```python
from build123d import *

# Parameters (mm, degrees)
ESQUISSE2_W                   = 150
ESQUISSE2_H                   = 150
BOSS_EXTRU_1_DEPTH            = 35
ESQUISSE3_R                   = 42.75
ENL_V_MAT_EXTRU_2_DEPTH       = 40
ESQUISSE5_R                   = 6
ENL_V_MAT_EXTRU_3_DEPTH       = 40
ESQUISSE6_R                   = 9.5
ENL_V_MAT_EXTRU_4_DEPTH       = 13
ESQUISSE7_R                   = 5.25
ENL_V_MAT_EXTRU_5_DEPTH       = 40
ESQUISSE8_R                   = 8.5
ENL_V_MAT_EXTRU_6_DEPTH       = 11
ESQUISSE9_R                   = 4.25
ENL_V_MAT_EXTRU_7_DEPTH       = 25
ENL_V_MAT_EXTRU_8_DEPTH       = 1
ENL_V_MAT_EXTRU_8_DEPTH_BACK  = 36
ENL_V_MAT_EXTRU_12_DEPTH      = 1
ENL_V_MAT_EXTRU_12_DEPTH_BACK = 36
ENL_V_MAT_EXTRU_13_DEPTH      = 1
ENL_V_MAT_EXTRU_13_DEPTH_BACK = 36
ENL_V_MAT_EXTRU_14_DEPTH      = 1
ENL_V_MAT_EXTRU_14_DEPTH_BACK = 36
CONG_1_R                      = 10
CONG_2_R                      = 10
CONG_3_R                      = 10
CONG_4_R                      = 10
CONG_5_R                      = 2


with BuildPart() as part:
    # Esquisse2 → Boss.-Extru.1 (new body)
    with BuildSketch(Plane.XY):
        with Locations((-75, 75)):
            Rectangle(ESQUISSE2_W, ESQUISSE2_H)
    extrude(amount=BOSS_EXTRU_1_DEPTH)

    # Esquisse3 → Enlèv. mat.-Extru.2 (cut)
    with BuildSketch(Plane.XY.offset(35)):
        with Locations((-75, 75)):
            Circle(ESQUISSE3_R)
    extrude(amount=-ENL_V_MAT_EXTRU_2_DEPTH, mode=Mode.SUBTRACT)

    # Esquisse5 → Enlèv. mat.-Extru.3 (cut)
    with BuildSketch(Plane.XY.offset(35)):
        with Locations((-28.5, 101.5)):
            Circle(ESQUISSE5_R)
        with Locations((-28.5, 48.5)):
            Circle(ESQUISSE5_R)
        with Locations((-121.5, 48.5)):
            Circle(ESQUISSE5_R)
        with Locations((-121.5, 101.5)):
            Circle(ESQUISSE5_R)
    extrude(amount=-ENL_V_MAT_EXTRU_3_DEPTH, mode=Mode.SUBTRACT)

    # Esquisse6 → Enlèv. mat.-Extru.4 (cut)
    with BuildSketch(Plane.XY.offset(35)):
        with Locations((-28.5, 101.5)):
            Circle(ESQUISSE6_R)
        with Locations((-28.5, 48.5)):
            Circle(ESQUISSE6_R)
        with Locations((-121.5, 48.5)):
            Circle(ESQUISSE6_R)
        with Locations((-121.5, 101.5)):
            Circle(ESQUISSE6_R)
    extrude(amount=-ENL_V_MAT_EXTRU_4_DEPTH, mode=Mode.SUBTRACT)

    # Esquisse7 → Enlèv. mat.-Extru.5 (cut)
    with BuildSketch(Plane.XY.offset(35)):
        with Locations((-11, 139)):
            Circle(ESQUISSE7_R)
        with Locations((-11, 11)):
            Circle(ESQUISSE7_R)
        with Locations((-139, 11)):
            Circle(ESQUISSE7_R)
        with Locations((-139, 139)):
            Circle(ESQUISSE7_R)
    extrude(amount=-ENL_V_MAT_EXTRU_5_DEPTH, mode=Mode.SUBTRACT)

    # Esquisse8 → Enlèv. mat.-Extru.6 (cut)
    with BuildSketch(Plane.XY.offset(35)):
        with Locations((-11, 139)):
            Circle(ESQUISSE8_R)
        with Locations((-11, 11)):
            Circle(ESQUISSE8_R)
        with Locations((-139, 11)):
            Circle(ESQUISSE8_R)
        with Locations((-139, 139)):
            Circle(ESQUISSE8_R)
    extrude(amount=-ENL_V_MAT_EXTRU_6_DEPTH, mode=Mode.SUBTRACT)

    # Esquisse9 → Enlèv. mat.-Extru.7 (cut)
    with BuildSketch(Plane(origin=(0, 150, 0), x_dir=(1, 0, 0), z_dir=(0, 1, 0))):
        with Locations(Location((-25, -25, 0), (0, 0, 270))):  # turned: the seam where the file's is
            Circle(ESQUISSE9_R)
        with Locations(Location((-125, -25, 0), (0, 0, 270))):  # turned: the seam where the file's is
            Circle(ESQUISSE9_R)
    extrude(amount=-ENL_V_MAT_EXTRU_7_DEPTH, mode=Mode.SUBTRACT)

    # Esquisse19 → Enlèv. mat.-Extru.8 (cut, two sides)
    with BuildSketch(Plane.XY.offset(35)) as enl_v_mat_extru_8_sk:
        with BuildLine():
            Line((206.944620495, 443.229107967), (0, 115))
            ThreePointArc((0, 115), (-11.557112298, 75), (0, 35))
            Line((0, 35), (206.944620495, -293.229107967))
            Line((206.944620495, -293.229107967), (982.986947353, -293.229107967))
            Line((982.986947353, -293.229107967), (982.986947353, 443.229107967))
            Line((982.986947353, 443.229107967), (206.944620495, 443.229107967))
        make_face()
    extrude(amount=ENL_V_MAT_EXTRU_8_DEPTH, mode=Mode.SUBTRACT)
    extrude(enl_v_mat_extru_8_sk.sketch, amount=-ENL_V_MAT_EXTRU_8_DEPTH_BACK, mode=Mode.SUBTRACT)

    # Esquisse22 → Enlèv. mat.-Extru.12 (cut, two sides)
    with BuildSketch(Plane.XY.offset(35)) as enl_v_mat_extru_12_sk:
        with BuildLine():
            Line((-443.229107967, -206.944620495), (-115, 0))
            ThreePointArc((-115, 0), (-75, 11.557112298), (-35, 0))
            Line((-35, 0), (293.229107967, -206.944620495))
            Line((293.229107967, -206.944620495), (293.229107967, -982.986947353))
            Line((293.229107967, -982.986947353), (-443.229107967, -982.986947353))
            Line((-443.229107967, -982.986947353), (-443.229107967, -206.944620495))
        make_face()
    extrude(amount=ENL_V_MAT_EXTRU_12_DEPTH, mode=Mode.SUBTRACT)
    extrude(enl_v_mat_extru_12_sk.sketch, amount=-ENL_V_MAT_EXTRU_12_DEPTH_BACK, mode=Mode.SUBTRACT)

    # Esquisse27 → Enlèv. mat.-Extru.13 (cut, two sides)
    with BuildSketch(Plane.XY.offset(35)) as enl_v_mat_extru_13_sk:
        with BuildLine():
            Line((-356.944620495, 443.229107967), (-150, 115))
            ThreePointArc((-150, 115), (-138.442887702, 75), (-150, 35))
            Line((-150, 35), (-356.944620495, -293.229107967))
            Line((-356.944620495, -293.229107967), (-1132.986947353, -293.229107967))
            Line((-1132.986947353, -293.229107967), (-1132.986947353, 443.229107967))
            Line((-1132.986947353, 443.229107967), (-356.944620495, 443.229107967))
        make_face()
    extrude(amount=ENL_V_MAT_EXTRU_13_DEPTH, mode=Mode.SUBTRACT)
    extrude(enl_v_mat_extru_13_sk.sketch, amount=-ENL_V_MAT_EXTRU_13_DEPTH_BACK, mode=Mode.SUBTRACT)

    # Esquisse28 → Enlèv. mat.-Extru.14 (cut, two sides)
    with BuildSketch(Plane.XY.offset(35)) as enl_v_mat_extru_14_sk:
        with BuildLine():
            Line((-443.229107967, 356.944620495), (-115, 150))
            ThreePointArc((-115, 150), (-75, 138.442887702), (-35, 150))
            Line((-35, 150), (293.229107967, 356.944620495))
            Line((293.229107967, 356.944620495), (293.229107967, 1132.986947353))
            Line((293.229107967, 1132.986947353), (-443.229107967, 1132.986947353))
            Line((-443.229107967, 1132.986947353), (-443.229107967, 356.944620495))
        make_face()
    extrude(amount=ENL_V_MAT_EXTRU_14_DEPTH, mode=Mode.SUBTRACT)
    extrude(enl_v_mat_extru_14_sk.sketch, amount=-ENL_V_MAT_EXTRU_14_DEPTH_BACK, mode=Mode.SUBTRACT)

    # Congé1
    cong_1_edges = [part.edges().sort_by_distance(p)[0] for p in [
        (0, 150, 17.5),
    ]]
    fillet(cong_1_edges, radius=CONG_1_R)

    # Congé2
    cong_2_edges = [part.edges().sort_by_distance(p)[0] for p in [
        (-150, 150, 17.5),
    ]]
    fillet(cong_2_edges, radius=CONG_2_R)

    # Congé3
    cong_3_edges = [part.edges().sort_by_distance(p)[0] for p in [
        (-150, 0, 17.5),
    ]]
    fillet(cong_3_edges, radius=CONG_3_R)

    # Congé4
    cong_4_edges = [part.edges().sort_by_distance(p)[0] for p in [
        (0, 0, 17.5),
    ]]
    fillet(cong_4_edges, radius=CONG_4_R)

    # Congé5
    cong_5_edges = [part.edges().sort_by_distance(p)[0] for p in [
        (-117.75, 75, 0),
    ]]
    fillet(cong_5_edges, radius=CONG_5_R)


solid = part.part
```
Verification items for the finished model (mm, model axes). A direction names the side the tool comes from. Coordinates: 2 decimals unless noted, no trailing zeros. Loops run counter-clockwise (first coordinate to the right, second up) from the corner with the lowest first, then second, coordinate; pieces in that order, holes last. Notation, with made-up numbers: (62.25, -39.5) -> (87.25, -39.5) arc R9 cw to (87.25, -33.5) -> close; hole circle Ø3 at (13, 65.25). An arc over 180 degrees is marked (long way). Put each result on its own line as item: value.
1. Gauge pin test, flat ends, axial feed: P1, Ø2, axis at y = 109.5, z = 24.5, coming from the -X side; P2, Ø3, axis at x = -118, y = 101.5, coming from the +Z side (1 decimal); P3, Ø13.5, axis at x = -139, y = 11, coming from the +Z side; P4, Ø2, axis at x = -105.5, z = 25.5, coming from the +Y side. Record the tip position at first contact, or that the pin passes through.
Result set:
P1: stops at x = -147.38
P2: passes through
P3: stops at z = 24
P4: stops at y = 145.38
2. Mould release check, pull along X, two halves, no side actions. Record for faces 4 (the face through (-131.15, 7.74, 29.58)), 5 (the face through (-75.591, 11.555, 17.745)), 6 (the face through (-23, 150, 17)), 7 (the face through (-3.01, 147.15, 17.74)): pulls with the +X half, pulls with the -X half, needs draft (parallel to the pull), parting line crosses it, or undercut.
Result set:
face 4: undercut
face 5: undercut
face 6: needs draft
face 7: pulls with the +X half
3. Section check C-C, the plane x = -125. Record the boundary of the cut face in (y, z), then the cut area to 3 significant figures.
Result set:
outline: (0, 0) -> (43.63, 0) -> (43.63, 22) -> (39.67, 22) -> (39.67, 35) -> (0, 35) -> close; (53.37, 0) -> (96.63, 0) -> (96.63, 22) -> (92.67, 22) -> (92.67, 35) -> (57.33, 35) -> (57.33, 22) -> (53.37, 22) -> close; (106.37, 0) -> (150, 0) -> (150, 20.75) -> (125, 20.75) -> (125, 29.25) -> (150, 29.25) -> (150, 35) -> (110.33, 35) -> (110.33, 22) -> (106.37, 22) -> close
area: 4,150 mm^2
4. Thickness scan on line 1 (Y direction, x = -28.5, z = 30.25); line 2 (Y direction, x = -121.5, z = 8); line 3 (Y direction, x = -90, z = 5). Record the ranges inside material, lowest first.
Result set:
line 1: y = 0 to 39, 58 to 92, 111 to 150
line 2: y = 0 to 42.5, 54.5 to 95.5, 107.5 to 150
line 3: y = 10.04 to 34.97, 115.03 to 139.96
5. Tool access check on faces 1 (the face through (-29.15, 137.68, 24.08)), 2 (the face through (-115, 49, 22)), 3 (the face through (-125.92, 105.56, 11.15)). Record the directions out of +Z, -Z, +X, -X, +Y, -Y that give a thin tool (end or side, any length) a straight path to the whole face; none if there is none.
Result set:
face 1: +Y
face 2: +Z
face 3: +Z, -Z
6. Section check B-B, the plane z = 15.5. Give the number of separate pieces and of enclosed holes in the cut face, then the cut area to 3 significant figures.
Result set:
separate pieces: 1
enclosed holes: 9
area: 13,400 mm^2
7. Section check A-A, the plane y = 75. Record the boundary of the cut face in (x, z), then the cut area to 3 significant figures.
Result set:
outline: (-138.44, 0) -> (-119.75, 0) arc R2 ccw to (-117.75, 2) -> (-117.75, 35) -> (-138.44, 35) -> close; (-32.25, 2) arc R2 ccw to (-30.25, 0) -> (-11.56, 0) -> (-11.56, 35) -> (-32.25, 35) -> close
area: 1,450 mm^2
